Model file for the job. Use its own axes, mm. A direction names the side the tool comes from. Give positions to 0.01 mm unless a question says otherwise; leave off trailing zeros. Order: outer loops, then holes, each group sorted by start corner. A loop starts at its lowest first (then second) coordinate and runs counter-clockwise, first axis right, second up. Notation, with made-up numbers: (57, 0) -> (112, 0) arc R11 cw to (112, 4) -> close; hole circle Ø7 at (27, 88). An arc over 180 degrees is marked (long way). Use CSV: the item, a comma, the result in double quotes. Start each with the question number.
1. Drop flat-ended pins along their axis: pin 1 (12.5 mm diameter, centred on x = -54.5, y = -21, fed in from -Z); pin 2 (0.5 mm diameter, centred on y = 30, z = 0.5, fed in from -X); pin 3 (0.8 mm diameter, centred on y = 13, z = 0.5, fed in from -X); pin 4 (3 mm diameter, centred on x = -14, y = 19.5, fed in from +Z). Give the stop position or say it passes through.
2. Cut at B-B on y = -25.5. List the corners of the cut face in (x, z), then the cut area to 3 significant figures.
3. Cut at A-A on z = 0.55. Give the number of separate pieces and of enclosed holes in the cut face, then the cut area to 3 significant figures.
4. Cut at C-C on x = 21. List the corners of the cut face in (y, z), then the cut area to 3 significant figures.
5. Pull direction Y, two halves, no side cores. Call faces 1 (the cylindrical face through (-50.48, 24.55, 1.81)), 2 (the flat face through (-38, 32.5, 1)), 3 (the flat face through (49, 22, 1)): released by +Y, released by -Y, zero draft, split by the parting line, or undercut.
6. Wall check: line 1 (Y direction, x = -32, z = 0.5); line 2 (Y direction, x = 10, z = 0.85); line 3 (X direction, y = 25, z = 0.95). Give the ranges that are in metal, low to high. Write a range as from..to.
7. 3-axis set-ups, long thin cutter, end or side, ignore diameter. For faces 4 (the flat face through (-41.896, 8, 1)), 5 (the flat face through (-33, 30, 1)), 6 (the flat face through (17, 11.5, 1)): which of +Z, -Z, +X, -X, +Y, -Y reach the whole face in a straight line?
```python
from build123d import *

# Parameters (mm, degrees)
P_IDAT_VYSUNUT_M1_DEPTH  = 3
SKICA3_W                 = 20.45
SKICA3_H                 = 3
ODEBRAT_VYSUNUT_M1_DEPTH = 1
ODEBRAT_VYSUNUT_M2_DEPTH = 1
ODEBRAT_VYSUNUT_M3_DEPTH = 1
SKICA6_W                 = 65
SKICA6_H                 = 21
ODEBRAT_VYSUNUT_M4_DEPTH = 69.302635381


with BuildPart() as part:
    # Skica2 → Přidat vysunutím1 (new body)
    with BuildSketch(Plane.XY):
        with BuildLine():
            Line((-60, 20.75), (-58.8, 20.75))
            ThreePointArc((-58.8, 20.75), (-50.347781356, 24.55), (-41.895562713, 20.75))
            Line((-41.895562713, 20.75), (-41.895562713, 16.25))
            Line((-41.895562713, 16.25), (-39.453287334, 16.25))
            ThreePointArc((-39.453287334, 16.25), (-39.047781356, 13.25), (-39.453287334, 10.25))
            Line((-39.453287334, 10.25), (-41.895562713, 10.25))
            Line((-41.895562713, 10.25), (-41.895562713, 5.75))
            ThreePointArc((-41.895562713, 5.75), (-50.347781356, 1.95), (-58.8, 5.75))
            Line((-58.8, 5.75), (-60, 5.75))
            Line((-60, 5.75), (-60, -32.5))
            Line((-60, -32.5), (60, -32.5))
            Line((60, -32.5), (60, 32.5))
            Line((60, 32.5), (-60, 32.5))
            Line((-60, 32.5), (-60, 20.75))
        make_face()
    extrude(amount=P_IDAT_VYSUNUT_M1_DEPTH)

    # Skica3 → Odebrat vysunutím1 (cut)
    with BuildSketch(Plane(origin=(0, 0, 0), x_dir=(-1, 0, 0), z_dir=(0, 0, -1))):
        with Locations((33.225, 30)):
            Rectangle(SKICA3_W, SKICA3_H)
    extrude(amount=-ODEBRAT_VYSUNUT_M1_DEPTH, mode=Mode.SUBTRACT)

    # Skica4 → Odebrat vysunutím2 (cut)
    with BuildSketch(Plane(origin=(0, 0, 0), x_dir=(-1, 0, 0), z_dir=(0, 0, -1))):
        Polygon((-59, 31.5), (-56, 31.5), (-56, -28.5), (43.45, -28.5), (43.45, -31.5), (-59, -31.5), align=None)
    extrude(amount=-ODEBRAT_VYSUNUT_M2_DEPTH, mode=Mode.SUBTRACT)

    # Skica5 → Odebrat vysunutím3 (cut)
    with BuildSketch(Plane(origin=(0, 0, 0), x_dir=(-1, 0, 0), z_dir=(0, 0, -1))):
        Polygon((60, 32.5), (48, 32.5), (48, 27.5), (44.45, 27.5), (44.45, -27.5), (48, -27.5), (48, -32.5), (60, -32.5), align=None)
    extrude(amount=-ODEBRAT_VYSUNUT_M3_DEPTH, mode=Mode.SUBTRACT)

    # Skica6 → Odebrat vysunutím4 (cut, through all)
    with BuildSketch(Plane(origin=(0, 0, 0), x_dir=(-1, 0, 0), z_dir=(0, 0, -1))):
        with Locations((-16.5, 22)):
            Rectangle(SKICA6_W, SKICA6_H)
    extrude(amount=-ODEBRAT_VYSUNUT_M4_DEPTH, mode=Mode.SUBTRACT)


solid = part.part
```
Verdict:
1,pin 1,"z = 1"
1,pin 2,"x = -48"
1,pin 3,"x = -39.07"
1,pin 4,"through"
2,outline,"(-60, 1) -> (-44.45, 1) -> (-44.45, 0) -> (56, 0) -> (56, 1) -> (59, 1) -> (59, 0) -> (60, 0) -> (60, 3) -> (-60, 3) -> close"
2,area,"341 mm^2"
3,separate pieces,"1"
3,enclosed holes,"2"
3,area,"4,850 mm^2"
4,outline,"(-32.5, 0) -> (-31.5, 0) -> (-31.5, 1) -> (-28.5, 1) -> (-28.5, 0) -> (11.5, 0) -> (11.5, 3) -> (-32.5, 3) -> close"
4,area,"129 mm^2"
5,face 1,"undercut"
5,face 2,"released by +Y"
5,face 3,"zero draft"
6,line 1,"-32.5..-31.5, -28.5..28.5, 31.5..32.5"
6,line 2,"-32.5..-31.5, -28.5..11.5"
6,line 3,"-44.45..-16, 49..56, 59..60"
7,face 4,"+Z, -Z, -X"
7,face 5,"-Z"
7,face 6,"+Z, -Z, +Y"
